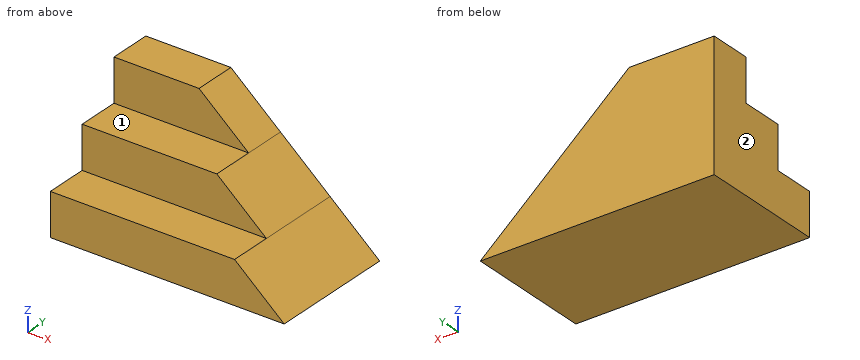
```python
from build123d import *

# Parameters (mm, degrees)
F1_DEPTH = 20
F2_DEPTH = 40
F3_DEPTH = 60


with BuildPart() as f1:
    # F0 (on Front) → F1 (new body)
    with BuildSketch(Plane.XZ):
        Polygon((0, 60), (0, 40), (63.333333, 40), (40, 60), align=None)
    extrude(amount=F1_DEPTH)

    # F0 (on Front) → F2 (join)
    with BuildSketch(Plane.XZ):
        Polygon((0, 40), (0, 20), (86.666667, 20), (63.333333, 40), align=None)
    extrude(amount=F2_DEPTH)

    # F0 (on Front) → F3 (join)
    with BuildSketch(Plane.XZ):
        Polygon((0, 20), (0, 0), (110, 0), (86.666667, 20), align=None)
    extrude(amount=F3_DEPTH)


solid = f1.part
```
Verification items for the finished model (mm, model axes). Face numbers are marked on the shaded views. A direction names the side the tool comes from. Round coordinates to 2 decimals unless told otherwise and drop trailing zeros. Order: outer loops, then holes, each group sorted by start corner. A loop starts at its lowest first (then second) coordinate and runs counter-clockwise, first axis right, second up. Notation, with made-up numbers: (62.25, -28.75) - (98.25, -28.75) arc R25 cw to (98.25, 7.25) - close; hole circle Ø6 at (-19, -7.75). An arc over 180 degrees is marked (long way). Use CSV: the item, a comma, the result in double quotes.
(1) Section check C-C on z = 18.5. Record the boundary of the cut face in (x, y).
Entries:
outline,"(0, -60) - (88.42, -60) - (88.42, 0) - (0, 0) - close"
(2) Section check B-B on x = 20.5. Record the boundary of the cut face in (y, z).
Entries:
outline,"(-60, 0) - (0, 0) - (0, 60) - (-20, 60) - (-20, 40) - (-40, 40) - (-40, 20) - (-60, 20) - close"
(3) Section check D-D on y = -26.5. Record the boundary of the cut face in (x, z), and give its area (3 significant figures).
Entries:
outline,"(0, 0) - (110, 0) - (63.33, 40) - (0, 40) - close"
area,"3,470 mm^2"
(4) Access from +Z, -Z, +X, -X, +Y, -Y to the whole of each face (thin tool, end or side, straight path). Record for the marked faces 1 and 2.
Entries:
face 1,"+Z, +X, -X, -Y"
face 2,"+Z, -Z, -X, +Y, -Y"
(5) Thickness scan on probe 1 along Y at (x, z) = (45, 52); probe 2 along Y at (x, z) = (26.5, 32.5); probe 3 along Z at (x, y) = (63.5, -54). Record the ranges inside material, lowest first. Write a range as from..to.
Entries:
probe 1,"-20..0"
probe 2,"-40..0"
probe 3,"0..20"
(6) Section check A-A on y = -4. Record the boundary of the cut face in (x, z), and give its area (3 significant figures).
Entries:
outline,"(0, 0) - (110, 0) - (40, 60) - (0, 60) - close"
area,"4,500 mm^2"
(7) Gauge pin test, flat ends, axial feed: pin 1 Ø10 at (x, y) = (42.5, -34.5) entering from +Z; pin 2 Ø1.5 at (x, y) = (93.5, -46) entering from +Z; pin 3 Ø2 at (y, z) = (-26.5, 17.5) entering from +X; pin 4 Ø8 at (x, z) = (78, 34.5) entering from +Y. Record the tip position at first contact, or that the pin passes through.
Entries:
pin 1,"z = 40"
pin 2,"z = 14.79"
pin 3,"x = 90.75"
pin 4,"through"
